from build123d import *

# Parameters (mm, degrees)
BOSS_EXTRUDE1_DEPTH = 7.5
SKETCH2_W           = 2
SKETCH2_H           = 9
BOSS_EXTRUDE2_DEPTH = 1
SKETCH3_W           = 38.42
SKETCH3_H           = 2
SKETCH3_W_2         = 86
SKETCH3_H_2         = 42
SKETCH3_W_3         = 80
SKETCH3_H_3         = 36
BOSS_EXTRUDE3_DEPTH = 8.5
SKETCH3_3_R         = 1.5
SKETCH3_3_W         = 47.58
SKETCH3_3_H         = 7.82
BOSS_EXTRUDE4_DEPTH = 2
FILLET1_R           = 3
FILLET2_R           = 2
SKETCH6_W           = 2
SKETCH6_H           = 7.82
BOSS_EXTRUDE5_DEPTH = 6.5
FILLET3_R           = 1
FILLET4_R           = 2


with BuildPart() as part:
    # Sketch1 → Boss-Extrude1 (new body)
    with BuildSketch(Plane.XY):
        Polygon((-2, -2), (-2, 4.59), (0, 4.59), (0, 0), (43.58, 0), (43.58, 18.18), (0, 18.18), (0, 13.59), (-2, 13.59), (-2, 20.18), (45.58, 20.18), (45.58, -2), align=None)
    extrude(amount=BOSS_EXTRUDE1_DEPTH)

    # Sketch2 → Boss-Extrude2 (add)
    with BuildSketch(Plane(origin=(0, 0, 0), x_dir=(-1, 0, 0), z_dir=(0, 0, -1))):
        with Locations((1, 9.09)):
            Rectangle(SKETCH2_W, SKETCH2_H)
        Polygon((0, 4.59), (0, 13.59), (0, 14.68), (-43.58, 14.68), (-43.58, 3.5), (0, 3.5), align=None)
        Polygon((2, 13.59), (2, 20.18), (-45.58, 20.18), (-45.58, -2), (2, -2), (2, 4.59), (0, 4.59), (0, 3.5), (0, 0), (-43.58, 0), (-43.58, 3.5), (-43.58, 14.68), (-43.58, 18.18), (0, 18.18), (0, 14.68), (0, 13.59), align=None)
    extrude(amount=BOSS_EXTRUDE2_DEPTH)

    # Sketch3 → Boss-Extrude3 (add)
    with BuildSketch(Plane(origin=(0, 0, -1), x_dir=(-1, 0, 0), z_dir=(0, 0, -1))):
        with Locations((-64.79, -1)):
            Rectangle(SKETCH3_W, SKETCH3_H)
        with Locations((-41, 49)):
            Rectangle(SKETCH3_W_2, SKETCH3_H_2)
        with Locations((-41, 49)):
            Rectangle(SKETCH3_W_3, SKETCH3_H_3, mode=Mode.SUBTRACT)
    extrude(amount=-BOSS_EXTRUDE3_DEPTH)

    # Sketch3<3> → Boss-Extrude4 (add)
    with BuildSketch(Plane(origin=(0, 0, -1), x_dir=(-1, 0, 0), z_dir=(0, 0, -1))):
        with BuildLine():
            Line((-6.854101966, 31), (-1, 31))
            Line((-1, 31), (-1, 37.741657387))
            ThreePointArc((-1, 37.741657387), (-6.897772597, 36.950447657), (-6.854101966, 31))
        make_face()
        with Locations((-3.5, 34)):
            Circle(SKETCH3_3_R, mode=Mode.SUBTRACT)
        with BuildLine():
            ThreePointArc((-6.854101966, 67), (-6.897772597, 61.049552343), (-1, 60.258342613))
            Line((-1, 60.258342613), (-1, 67))
            Line((-1, 67), (-6.854101966, 67))
        make_face()
        with Locations((-3.5, 64)):
            Circle(SKETCH3_3_R, mode=Mode.SUBTRACT)
        with BuildLine():
            Line((-81, 67), (-81, 60.258342613))
            ThreePointArc((-81, 60.258342613), (-75.102227403, 61.049552343), (-75.145898034, 67))
            Line((-75.145898034, 67), (-81, 67))
        make_face()
        with Locations((-78.5, 64)):
            Circle(SKETCH3_3_R, mode=Mode.SUBTRACT)
        with BuildLine():
            Line((-81, 31), (-75.145898034, 31))
            ThreePointArc((-75.145898034, 31), (-75.102227403, 36.950447657), (-81, 37.741657387))
            Line((-81, 37.741657387), (-81, 31))
        make_face()
        with Locations((-78.5, 34)):
            Circle(SKETCH3_3_R, mode=Mode.SUBTRACT)
        with Locations((-21.79, 24.09)):
            Rectangle(SKETCH3_3_W, SKETCH3_3_H)
        Polygon((-84, 0), (-45.58, 0), (-45.58, 20.18), (-45.58, 28), (-84, 28), align=None)
    extrude(amount=-BOSS_EXTRUDE4_DEPTH)

    # Fillet1
    fillet1_edges = [part.edges().sort_by_distance(p)[0] for p in [
        (1, 37.741657387, 0),
        (6.854101966, 31, 0),
        (6.854101966, 67, 0),
        (1, 60.258342613, 0),
        (81, 60.258342613, 0),
        (75.145898034, 67, 0),
        (75.145898034, 31, 0),
        (81, 37.741657387, 0),
    ]]
    fillet(fillet1_edges, radius=FILLET1_R)

    # Fillet2
    fillet2_edges = [part.edges().sort_by_distance(p)[0] for p in [
        (-2, -2, 3.25),
        (-2, 70, 3.25),
        (84, 70, 3.25),
    ]]
    fillet(fillet2_edges, radius=FILLET2_R)

    # Sketch6 → Boss-Extrude5 (add)
    with BuildSketch(Plane.XY.offset(1)):
        with Locations((44.58, 24.09)):
            Rectangle(SKETCH6_W, SKETCH6_H)
    extrude(amount=BOSS_EXTRUDE5_DEPTH)

    # Fillet3
    fillet3_edges = [part.edges().sort_by_distance(p)[0] for p in [
        (-1, 4.59, 0),
        (-1, 13.59, 0),
    ]]
    fillet(fillet3_edges, radius=FILLET3_R)

    # Fillet4
    fillet4_edges = [part.edges().sort_by_distance(p)[0] for p in [
        (-1, 4.59, 7.5),
        (-1, 13.59, 7.5),
    ]]
    fillet(fillet4_edges, radius=FILLET4_R)


solid = part.part
Here's how the part is built. I have some questions about the finished solid (model axes, mm). A direction names the side the tool comes from. Round coordinates to 2 decimals unless told otherwise and drop trailing zeros. Write each loop counter-clockwise with the first axis right and the second up, starting at its lowest first coordinate (ties: lowest second). Pieces come first, ordered by that corner, then holes. Notation, with made-up numbers: (56.5, -27) -> (77.5, -27) arc R16 cw to (77.5, -18) -> close; hole circle Ø11 at (68.5, -34.75). An arc over 180 degrees is marked (long way). One line per item, written item: value.
1) Suppose I cut it at D-D on x = 40. List the corners of the cut face in (y, z) for me.
Filled sheet:
outline: (-2, -1) -> (0, -1) -> (0, 7.5) -> (-2, 7.5) -> close; (3.5, -1) -> (14.68, -1) -> (14.68, 0) -> (3.5, 0) -> close; (18.18, -1) -> (31, -1) -> (31, 7.5) -> (28, 7.5) -> (28, 1) -> (20.18, 1) -> (20.18, 7.5) -> (18.18, 7.5) -> close; (67, -1) -> (70, -1) -> (70, 7.5) -> (67, 7.5) -> close
2) I'm going to push flat-ended pins straight in: pin 1 Ø8.5 at (x, y) = (68, 11) entering from +Z; pin 2 Ø3 at (y, z) = (4, 4) entering from +X. Where does each tip first touch, or does it pass through?
Filled sheet:
pin 1: stops at z = 1
pin 2: stops at x = 45.58
3) If I drill on line 1 (Y direction, x = 42, z = 2.5); line 2 (Y direction, x = 46.5, z = 6); line 3 (Y direction, x = 3.5, z = 0.55), over which ranges is the centre line in solid material (lowest first)? Write a range as [from, to].
Filled sheet:
line 1: y = [-2, 0], [18.18, 20.18], [28, 31], [67, 70]
line 2: y = [-2, 0], [28, 31], [67, 70]
line 3: y = [-2, 0], [18.18, 32.5], [35.5, 38.53], [59.47, 62.5], [65.5, 70]
4) We'd pull the mould along X, two halves only. Please class faces 5 (the face through (-1, 4.59, 3)), 6 (the face through (-1.43, -1.4, 3.31)), 7 (the face through (77, 35, 1)): released by +X, released by -X, zero draft, split by the parting line, or undercut.
Filled sheet:
face 5: zero draft
face 6: released by -X
face 7: undercut
5) Suppose I cut it at B-B on x = 55. List the corners of the cut face in (y, z) for me, plus the area to 3 significant figures.
Filled sheet:
outline: (-2, -1) -> (31, -1) -> (31, 7.5) -> (28, 7.5) -> (28, 1) -> (0, 1) -> (0, 7.5) -> (-2, 7.5) -> close; (67, -1) -> (70, -1) -> (70, 7.5) -> (67, 7.5) -> close
area: 124 mm2
6) Suppose I cut it at C-C on y = 37.5. List the corners of the cut face in (x, z) for me.
Filled sheet:
outline: (-2, -1) -> (6.33, -1) -> (6.33, 1) -> (1, 1) -> (1, 7.5) -> (-2, 7.5) -> close; (75.67, -1) -> (84, -1) -> (84, 7.5) -> (81, 7.5) -> (81, 1) -> (75.67, 1) -> close
7) Suppose I cut it at A-A on z = 3.25. List the corners of the cut face in (x, y) for me.
Filled sheet:
outline: (-2, 0) arc R2 ccw to (0, -2) -> (84, -2) -> (84, 0) -> (45.58, 0) -> (45.58, 28) -> (84, 28) -> (84, 68) arc R2 ccw to (82, 70) -> (0, 70) arc R2 ccw to (-2, 68) -> (-2, 28) -> (43.58, 28) -> (43.58, 20.18) -> (-2, 20.18) -> (-2, 13.59) -> (0, 13.59) -> (0, 18.18) -> (43.58, 18.18) -> (43.58, 0) -> (0, 0) -> (0, 4.59) -> (-2, 4.59) -> close; hole (1, 31) -> (81, 31) -> (81, 67) -> (1, 67) -> close
8) For faces 1 (the face through (81, 49, 4)), 2 (the face through (-1, 13.59, 3)), 3 (the face through (8.86, 31.9, 0.01)), 4 (the face through (45.58, 14, 4)), which set-ups out of +Z, -Z, +X, -X, +Y, -Y let a thin tool reach every point of the face, with its end or its side?
Filled sheet:
face 1: +Z
face 2: +Z, -X
face 3: +Z, -Z
face 4: +Z, +X
